For this review, take the finished solid that the model builds, in its own axes (mm). A direction names the side the tool comes from. Coordinates: 2 decimals unless noted, no trailing zeros. Order: outer loops, then holes, each group sorted by start corner. A loop starts at its lowest first (then second) coordinate and runs counter-clockwise, first axis right, second up. Notation, with made-up numbers: M 11,-32.5 L 16,-32.5 A23 ccw 16,-2.5 Z; hole C 52,74 d9. An arc over 180 degrees is marked long. Use CSV: the item, a comma, the result in double quotes.
```python
from build123d import *

# Parameters (mm, degrees)
F0_R     = 8.119987
F1_DEPTH = 8.89
F4_R     = 4.141817
F5_DEPTH = 5.9182
F6_R     = 4.114136
F7_DEPTH = 5.588
F8_DEPTH = 8.382
F9_DEPTH = 8.6106


with BuildPart() as f1:
    # F0 (on Right) → F1 (new body)
    with BuildSketch(Plane.YZ):
        with BuildLine():
            Line((-38.991049, -16.499758), (0, -16.499758))
            Line((0, -16.499758), (38.991049, -16.499758))
            ThreePointArc((38.991049, -16.499758), (55.02992, -0.460887), (38.991049, 15.577984))
            Line((38.991049, 15.577984), (-38.991049, 15.577984))
            ThreePointArc((-38.991049, 15.577984), (-55.02992, -0.460887), (-38.991049, -16.499758))
        make_face()
        with Locations((-38.991049, -0.460887)):
            Circle(F0_R, mode=Mode.SUBTRACT)
        with Locations((38.991049, -0.460887)):
            Circle(F0_R, mode=Mode.SUBTRACT)
    extrude(amount=F1_DEPTH)

    # F4 (on offset) → F5 (join)
    with BuildSketch(Plane.XZ.offset(21.082)):
        with BuildLine():
            Line((0, -8.503367), (0, 8.564635))
            Line((0, 8.564635), (-23.786137, 8.564635))
            ThreePointArc((-23.786137, 8.564635), (-32.24461, -0.007005), (-23.710525, -8.503367))
            Line((-23.710525, -8.503367), (0, -8.503367))
        make_face()
        with Locations((-23.710525, 0.030801)):
            Circle(F4_R, mode=Mode.SUBTRACT)
    extrude(amount=F5_DEPTH)

    # F6 (on Front) → F7 (join)
    with BuildSketch(Plane.XZ):
        with BuildLine():
            Line((0, -8.482178), (0, 8.645641))
            Line((0, 8.645641), (-23.690745, 8.645641))
            ThreePointArc((-23.690745, 8.645641), (-32.255356, -0.029298), (-23.47151, -8.482178))
            Line((-23.47151, -8.482178), (0, -8.482178))
        make_face()
        with Locations((-23.690745, 0.080328)):
            Circle(F6_R, mode=Mode.SUBTRACT)
    extrude(amount=-F7_DEPTH)

    # F3 (on Top) → F8 (join)
    with BuildSketch(Plane.XY):
        with BuildLine():
            ThreePointArc((-11.469169, 0), (-4.959083, -10.488037), (-11.284814, -21.088285))
            Line((-11.284814, -21.088285), (0, -21.167291))
            Line((0, -21.167291), (0, 0))
            Line((0, 0), (-11.469169, 0))
        make_face()
    extrude(amount=F8_DEPTH)

    # F8_face (on face) → F9 (join)
    with BuildSketch(Plane(origin=(-3.631356, -10.506783, 0), x_dir=(1, 0, 0), z_dir=(0, 0, -1))):
        with BuildLine():
            Line((-7.837812, -10.506783), (3.631356, -10.506783))
            Line((3.631356, -10.506783), (3.631356, 10.575217))
            Line((3.631356, 10.575217), (-7.641576, 10.575217))
            ThreePointArc((-7.641576, 10.575217), (-1.327787, -0.025466), (-7.837812, -10.506783))
        make_face()
    extrude(amount=F9_DEPTH)


solid = f1.part
```
Item 1: To check wall thickness, follow line 1 along Z through (x, y) = (-17.5, -22); line 2 along X through (y, z) = (15, -4); line 3 along Y through (x, z) = (-22, 7.5). State the ranges of each line that lie inside material, in increasing order. Write a range as [from, to].
Solutions:
line 1,"[-8.5, 8.56]"
line 2,"[0, 8.89]"
line 3,"[-27, -21.08], [0, 5.59]"
Item 2: Draft analysis for pull direction Y (two halves, no side actions). For faces 1 (the face through (4.383, 55.026, -0.814)), 2 (the face through (-20, -21.082, 4)), 3 (the face through (-12, -24, 8.565)), state which applies: released by +Y, released by -Y, zero draft, split by the parting line, or undercut.
Solutions:
face 1,"released by +Y"
face 2,"undercut"
face 3,"zero draft"
Item 3: Clearance check with flat-ended pins moving along their axes: pin 1 Ø3 at (x, y) = (-17.5, 3) entering from +Z; pin 2 Ø12 at (y, z) = (-29, -11.5) entering from -X; pin 3 Ø5.5 at (x, y) = (-5, -11.5) entering from -Z. State where each tip first meets the part, or that it passes through.
Solutions:
pin 1,"z = 8.65"
pin 2,"x = -29.9"
pin 3,"z = -8.61"
Item 4: Add section A-A on x = -3.5. State the section outline as (y, z) points.
Solutions:
outline,"M -27,-8.5 L -21.08,-8.5 L -21.08,-8.61 L 0,-8.61 L 0,-8.48 L 5.59,-8.48 L 5.59,8.65 L 0,8.65 L 0,8.38 L -21.08,8.38 L -21.08,8.56 L -27,8.56 Z"
Item 5: For faces 4 (the face through (-13, 5.588, 0)), 5 (the face through (-12, 3, -8.482)), 6 (the face through (-12, 3, 8.646)), 7 (the face through (-3, -10, 8.382)), 8 (the face through (-32.243, -24, 0.18)), list the 3-axis set-ups (+Z, -Z, +X, -X, +Y, -Y) from which the entire face can be reached by the end or side of a thin tool; tool diameter is ignored.
Solutions:
face 4,"+Z, -Z, -X, +Y"
face 5,"-Z, -X, +Y"
face 6,"+Z, -X, +Y, -Y"
face 7,"+Z, -X"
face 8,"-X, -Y"
Item 6: Add section B-B on y = -45. State the section outline as (x, z) points, and give its area (3 significant figures).
Solutions:
outline,"M 0,-15.33 L 8.89,-15.33 L 8.89,-5.92 L 0,-5.92 Z; M 0,5 L 8.89,5 L 8.89,14.41 L 0,14.41 Z"
area,"167 mm^2"
Item 7: Add section C-C on z = -6. State the section outline as (x, y) points, and give its area (3 significant figures).
Solutions:
outline,"M -29.75,-27 L 0,-27 L 0,-33.05 L 8.89,-33.05 L 8.89,33.05 L 0,33.05 L 0,5.59 L -29.72,5.59 L -29.72,0 L -11.47,0 A11.87 cw -11.27,-21.08 L -29.75,-21.08 Z; M 0,-54.04 L 8.89,-54.04 L 8.89,-44.93 L 0,-44.93 Z; M 0,44.93 L 8.89,44.93 L 8.89,54.04 L 0,54.04 Z"
area,"1,240 mm^2"
Item 8: Add section D-D on x = -21. State the section outline as (y, z) points.
Solutions:
outline,"M -27,-8.5 L -21.08,-8.5 L -21.08,-3.1 L -27,-3.1 Z; M -27,3.16 L -21.08,3.16 L -21.08,8.56 L -27,8.56 Z; M 0,-8.48 L 5.59,-8.48 L 5.59,-3.03 L 0,-3.03 Z; M 0,3.19 L 5.59,3.19 L 5.59,8.65 L 0,8.65 Z"
